The figure shows three views and two pictorial views of one solid part (mm, origin at its lowest corner). Answer the questions. A direction names the side the tool comes from. Give positions to 0.01 mm unless a question says otherwise; leave off trailing zeros. Order: outer loops, then holes, each group sorted by start corner. A loop starts at its lowest first (then second) coordinate and runs counter-clockwise, first axis right, second up. Notation, with made-up numbers: (30, 15) - (43, 15) arc R20 ccw to (43, 40) - close; hole circle Ø11 at (-30, 59). An arc over 180 degrees is marked (long way). Answer as CSV lines item,"result". Start each with the question number.
1. Which of the six approach directions +Z, -Z, +X, -X, +Y, -Y give full straight-line access (tool end or side, diameter ignored) to the marked faces 4 and 5?
2. Section A-A on z = 77.5 is taken. Give the vertices of the cut face in (x, y) (1 decimal).
3. Determine the mould class of the marked faces 1, 2 and 3 for opening direction Z: +Z half, -Z half, draft (parallel to the pull), parting line (faces both ways), or undercut.
4. Section D-D on x = 124.5 is taken. Give the vertices of the cut face in (y, z), and give its area (3 significant figures).
5. Consider line 1 along X through (y, z) = (9.25, 77); line 2 along Y through (x, z) = (65.5, 64) (1 decimal); line 3 along X through (y, z) = (0.8, 77.5). Determine where each line is inside the solid, lowest interval first. Write a range as [from, to].
6. Flat-ended cylindrical pins translate along their axes: pin 1 (1.5 mm diameter, centred on y = 7.5, z = 108.5, fed in from -X); pin 2 (23.5 mm diameter, centred on x = 69.17, z = 91.93, fed in from +Y); pin 3 (3 mm diameter, centred on x = 100, y = 8, fed in from +Z); pin 4 (16.5 mm diameter, centred on x = 85.83, z = 63.07, fed in from +Y). Find the tip coordinate at first contact, or state that the pin passes through.
7. Section C-C on x = 58 is taken. Give the vertices of the cut face in (y, z) (1 decimal).
8. Section B-B on y = 14 is taken. Give the vertices of the cut face in (x, z) (1 decimal).
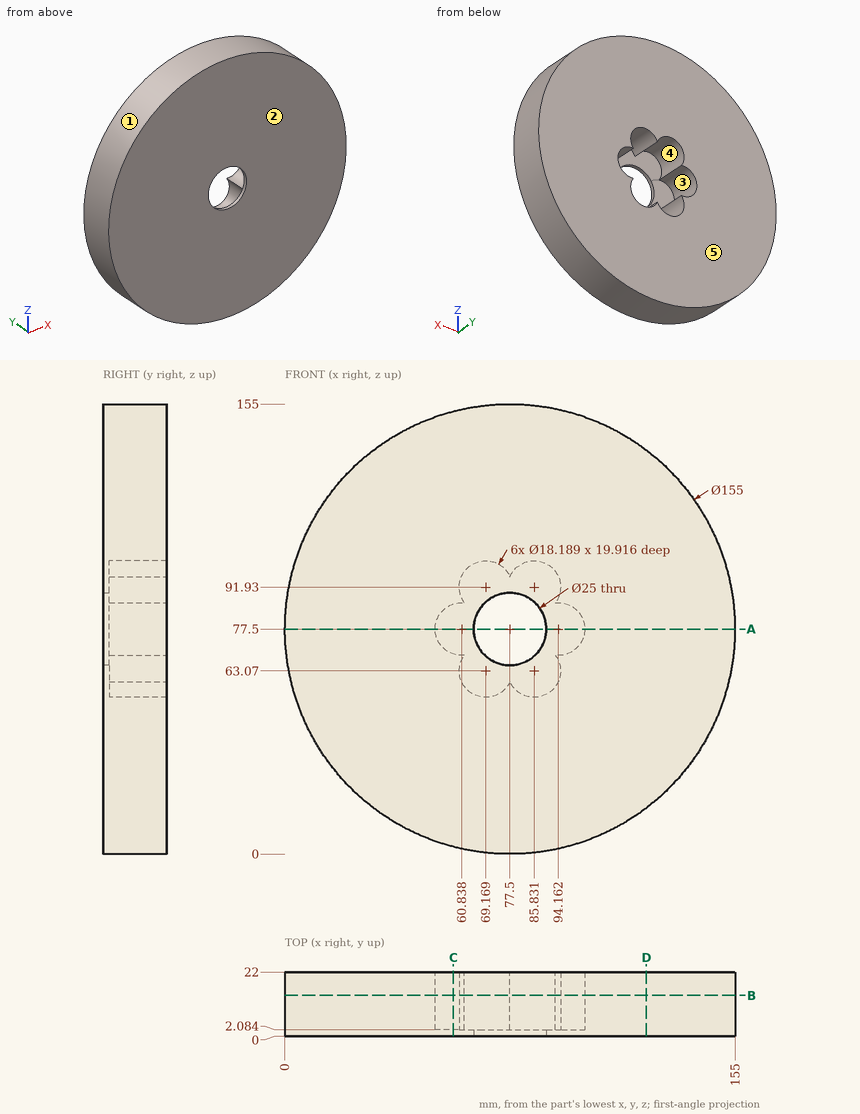
Checks:
1,face 4,"+Y"
1,face 5,"+Z, -Z, +X, -X, +Y"
2,outline,"(0, 0) - (65, 0) - (65, 2.1) - (51.7, 2.1) - (51.7, 22) - (0, 22) - close; (90, 0) - (155, 0) - (155, 22) - (103.3, 22) - (103.3, 2.1) - (90, 2.1) - close"
3,face 1,"parting line"
3,face 2,"draft"
3,face 3,"undercut"
4,outline,"(0, 15.88) - (22, 15.88) - (22, 139.12) - (0, 139.12) - close"
4,area,"2,710 mm²"
5,line 1,"x = [0, 51.76], [103.24, 155]"
5,line 2,"y = [0, 2.1]"
5,line 3,"x = [0, 65], [90, 155]"
6,pin 1,"stops at x = 6.15"
6,pin 2,"stops at y = 22"
6,pin 3,"stops at z = 152.1"
6,pin 4,"stops at y = 2.08"
7,outline,"(0, 2.5) - (22, 2.5) - (22, 68.9) - (2.1, 68.9) - (2.1, 86.1) - (22, 86.1) - (22, 152.5) - (0, 152.5) - close"
8,outline,"circle Ø155 at (77.5, 77.5); hole (61.8, 68.5) arc R9.1 ccw (long way) to (77.5, 59.4) arc R9.1 ccw (long way) to (93.2, 68.5) arc R9.1 ccw (long way) to (93.2, 86.5) arc R9.1 ccw (long way) to (77.5, 95.6) arc R9.1 ccw (long way) to (61.8, 86.5) arc R9.1 ccw (long way) to start"
